The listing builds one solid part. Answer for the finished solid, in the listing's coordinates (mm). A direction names the side the tool comes from. Round coordinates to 2 decimals unless told otherwise and drop trailing zeros. Write each loop counter-clockwise with the first axis right and the second up, starting at its lowest first coordinate (ties: lowest second). Pieces come first, ordered by that corner, then holes.
(1) Each of these flat-tipped pins is pushed along its axis until it touches: pin 1 Ø1.5 at (x, y) = (-14, 2.5) entering from +Z; pin 2 Ø1.6 at (x, z) = (14, 0) entering from +Y; pin 3 Ø2 at (x, z) = (-5.5, 2.5) entering from -Y; pin 4 Ø2 at (x, z) = (-13, 12.5) entering from -Y. Where does it stop, or does it pass through?
(2) A cutting plane is placed at B-B, the plane x = 0. Give the vertices of the cut face in (y, z), and give its area (3 significant figures).
(3) A cutting plane is placed at D-D, the plane z = -12.75. Give the vertices of the cut face in (x, y).
(4) Find the intervals of material crossed by probe 1 along Z at (x, y) = (-12.5, 1); probe 2 along X at (y, z) = (9.5, 2); probe 3 along Z at (x, y) = (10.5, 2.25), in increasing order.
(5) A cutting plane is placed at C-C, the plane z = 0. Give the vertices of the cut face in (x, y).
(6) For faces 1 (the face through (-7.81, 2.86, 1.73)), 2 (the face through (-7, 6, -12)), 3 (the face through (12, 11, -13)), determine the directions among +Z, -Z, +X, -X, +Y, -Y from which every point of the face is accessible in a straight line to the end or side of a thin tool.
(7) A cutting plane is placed at A-A, the plane y = 9.5. Give the vertices of the cut face in (x, z), and give its area (3 significant figures).
(8) The mould has two halves that part along X. Classify faces 4 (the face through (7, 6, -12)), 5 (the face through (-8, 0, 4)): +X half, -X half, draft (parallel to the pull), parting line (faces both ways), or undercut.
from build123d import *

# Parameters (mm, degrees)
SKETCH1_R           = 17.5
BOSS_EXTRUDE1_DEPTH = 11
SKETCH2_R           = 19.5
BOSS_EXTRUDE2_DEPTH = 1.5
SKETCH3_R           = 10.5
CUT_EXTRUDE1_DEPTH  = 5.2
SKETCH4_R           = 8.5
CUT_EXTRUDE2_DEPTH  = 1.5
CUT_EXTRUDE4_REACH  = 32.278
SKETCH7_R           = 8
SKETCH9_R           = 2.7
CUT_EXTRUDE5_DEPTH  = 6
SKETCH10_R          = 2.7
CUT_EXTRUDE6_DEPTH  = 6.5


with BuildPart() as part:
    # Sketch1 → Boss-Extrude1 (new body)
    with BuildSketch(Plane(origin=(0, 0, 0), x_dir=(1, 0, 0), z_dir=(0, 1, 0))):
        with Locations(Location((0, 0, 0), (0, 0, 270))):
            Circle(SKETCH1_R)
    extrude(amount=BOSS_EXTRUDE1_DEPTH)

    # Sketch2 → Boss-Extrude2 (add)
    with BuildSketch(Plane(origin=(0, 11, 0), x_dir=(1, 0, 0), z_dir=(0, 1, 0))):
        with Locations(Location((0, 0, 0), (0, 0, 270))):
            Circle(SKETCH2_R)
    extrude(amount=BOSS_EXTRUDE2_DEPTH)

    # Sketch3 → Cut-Extrude1 (cut)
    with BuildSketch(Plane(origin=(0, 12.5, 0), x_dir=(1, 0, 0), z_dir=(0, 1, 0))):
        with Locations(Location((0, 0, 0), (0, 0, 270))):
            Circle(SKETCH3_R)
    extrude(amount=-CUT_EXTRUDE1_DEPTH, mode=Mode.SUBTRACT)

    # Sketch4 → Cut-Extrude2 (cut)
    with BuildSketch(Plane(origin=(0, 7.3, 0), x_dir=(1, 0, 0), z_dir=(0, 1, 0))):
        with Locations(Location((0, 0, 0), (0, 0, 270))):
            Circle(SKETCH4_R)
    extrude(amount=-CUT_EXTRUDE2_DEPTH, mode=Mode.SUBTRACT)

    # Sketch7 → Cut-Extrude4 (cut, up to next)
    with BuildSketch(Plane.XZ, mode=Mode.PRIVATE) as cut_extrude4_sk1:
        with Locations(Location((0, 0, 0), (0, 0, 270))):
            Circle(SKETCH7_R)
    cut_extrude4_tool1 = extrude(cut_extrude4_sk1.sketch, amount=-CUT_EXTRUDE4_REACH, mode=Mode.PRIVATE) & part.part
    add(cut_extrude4_tool1.solids().sort_by_distance((0, 0, 0))[0], mode=Mode.SUBTRACT)

    # Sketch9 → Cut-Extrude5 (cut)
    with BuildSketch(Plane.XZ):
        with Locations(Location((0, 12.75, 0), (0, 0, 270))):
            Circle(SKETCH9_R)
        with Locations(Location((11.041823898, 6.375, 0), (0, 0, 270))):
            Circle(SKETCH9_R)
        with Locations(Location((11.041823898, -6.375, 0), (0, 0, 270))):
            Circle(SKETCH9_R)
        with Locations(Location((0, -12.75, 0), (0, 0, 270))):
            Circle(SKETCH9_R)
        with Locations(Location((-11.041823898, -6.375, 0), (0, 0, 270))):
            Circle(SKETCH9_R)
        with Locations(Location((-11.041823898, 6.375, 0), (0, 0, 270))):
            Circle(SKETCH9_R)
    extrude(amount=-CUT_EXTRUDE5_DEPTH, mode=Mode.SUBTRACT)

    # Sketch10 → Cut-Extrude6 (cut)
    with BuildSketch(Plane(origin=(0, 12.5, 0), x_dir=(1, 0, 0), z_dir=(0, 1, 0))):
        with Locations(Location((14, 0, 0), (0, 0, 270))):
            Circle(SKETCH10_R)
        with Locations(Location((7, -12.124355653, 0), (0, 0, 270))):
            Circle(SKETCH10_R)
        with Locations(Location((-7, -12.124355653, 0), (0, 0, 270))):
            Circle(SKETCH10_R)
        with Locations(Location((-14, 0, 0), (0, 0, 270))):
            Circle(SKETCH10_R)
        with Locations(Location((-7, 12.124355653, 0), (0, 0, 270))):
            Circle(SKETCH10_R)
        with Locations(Location((7, 12.124355653, 0), (0, 0, 270))):
            Circle(SKETCH10_R)
    extrude(amount=-CUT_EXTRUDE6_DEPTH, mode=Mode.SUBTRACT)


solid = part.part
Solutions:
1. pin 1: stops at z = 11.43
1. pin 2: stops at y = 6
1. pin 3: passes through
1. pin 4: stops at y = 0
2. outline: (0, -17.5) - (11, -17.5) - (11, -19.5) - (12.5, -19.5) - (12.5, -10.5) - (7.3, -10.5) - (7.3, -8.5) - (5.8, -8.5) - (5.8, -8) - (0, -8) - (0, -10.05) - (6, -10.05) - (6, -15.45) - (0, -15.45) - close; (0, 8) - (5.8, 8) - (5.8, 8.5) - (7.3, 8.5) - (7.3, 10.5) - (12.5, 10.5) - (12.5, 19.5) - (11, 19.5) - (11, 17.5) - (0, 17.5) - (0, 15.45) - (6, 15.45) - (6, 10.05) - (0, 10.05) - close
2. area: 151 mm2
3. outline: (-14.75, 11) - (-11.99, 11) - (-11.99, 0) - (-2.7, 0) - (-2.7, 6) - (2.7, 6) - (2.7, 0) - (11.99, 0) - (11.99, 11) - (14.75, 11) - (14.75, 12.5) - (9.63, 12.5) - (9.63, 6) - (4.37, 6) - (4.37, 12.5) - (-4.37, 12.5) - (-4.37, 6) - (-9.63, 6) - (-9.63, 12.5) - (-14.75, 12.5) - close
4. probe 1: z = -12.25 to -8.65, -4.1 to 4.1, 8.65 to 12.25
4. probe 2: x = -17.39 to -15.81, -12.19 to -10.31, 10.31 to 12.19, 15.81 to 17.39
4. probe 3: z = -14 to -9.02, -3.73 to 3.73, 9.02 to 14
5. outline: (-19.5, 11) - (-17.5, 11) - (-17.5, 0) - (-8, 0) - (-8, 5.8) - (-8.5, 5.8) - (-8.5, 7.3) - (-10.5, 7.3) - (-10.5, 12.5) - (-11.3, 12.5) - (-11.3, 6) - (-16.7, 6) - (-16.7, 12.5) - (-19.5, 12.5) - close; (8, 0) - (17.5, 0) - (17.5, 11) - (19.5, 11) - (19.5, 12.5) - (16.7, 12.5) - (16.7, 6) - (11.3, 6) - (11.3, 12.5) - (10.5, 12.5) - (10.5, 7.3) - (8.5, 7.3) - (8.5, 5.8) - (8, 5.8) - close
6. face 1: +Y, -Y
6. face 2: +Y
6. face 3: -Y
7. outline: circle Ø35 at (0, 0); hole circle Ø5.4 at (-14, 0); hole circle Ø21 at (0, 0); hole circle Ø5.4 at (-7, -12.12); hole circle Ø5.4 at (-7, 12.12); hole circle Ø5.4 at (7, -12.12); hole circle Ø5.4 at (7, 12.12); hole circle Ø5.4 at (14, 0)
7. area: 478 mm2
8. face 4: undercut
8. face 5: draft
